```python
from build123d import *

# Parameters (mm, degrees)
SKETCH_1_W          = 20
SKETCH_1_H          = 60
EXTRUDE_1_DEPTH     = 240
SKETCH_2_W          = 14
SKETCH_2_H          = 54
CUT_EXTRUDE_1_DEPTH = 241
SKETCH_3_R          = 2
CUT_EXTRUDE_2_DEPTH = 240
SKETCH_4_R          = 3.05
SKETCH_4_R_2        = 2
CUT_EXTRUDE_3_DEPTH = 61


with BuildPart() as part:
    # 草图1 → 凸台-拉伸1 (new body)
    with BuildSketch(Plane.XY):
        with Locations((-26.616848502, -4.212119477)):
            Rectangle(SKETCH_1_W, SKETCH_1_H)
    extrude(amount=EXTRUDE_1_DEPTH)

    # 草图2 → 切除-拉伸1 (cut, through all)
    with BuildSketch(Plane.XY.offset(240)):
        with Locations((-26.616848502, -4.212119477)):
            Rectangle(SKETCH_2_W, SKETCH_2_H)
    extrude(amount=-CUT_EXTRUDE_1_DEPTH, mode=Mode.SUBTRACT)

    # 草图3 → 切除-拉伸2 (cut)
    with BuildSketch(Plane(origin=(-16.616848502, 0, 0), x_dir=(0, 0, -1), z_dir=(1, 0, 0))):
        with Locations((-220, 19.787880523)):
            Circle(SKETCH_3_R)
        with Locations((-20, 19.787880523)):
            Circle(SKETCH_3_R)
        with Locations((-181.67, 19.787880523)):
            Circle(SKETCH_3_R)
        with Locations((-220, -26.212119477)):
            Circle(SKETCH_3_R)
        with Locations((-181.67, -26.212119477)):
            Circle(SKETCH_3_R)
        with Locations((-20, -26.212119477)):
            Circle(SKETCH_3_R)
        with Locations((-58.33, -26.212119477)):
            Circle(SKETCH_3_R)
        with Locations((-58.33, 19.787880523)):
            Circle(SKETCH_3_R)
    extrude(amount=-CUT_EXTRUDE_2_DEPTH, mode=Mode.SUBTRACT)

    # 草图4 → 切除-拉伸3 (cut, through all)
    with BuildSketch(Plane(origin=(0, 25.787880523, 0), x_dir=(1, 0, 0), z_dir=(0, 1, 0))):
        with Locations((-26.616848502, -220)):
            Circle(SKETCH_4_R)
        with Locations((-26.616848502, -190)):
            Circle(SKETCH_4_R_2)
        with Locations((-26.616848502, -135)):
            Circle(SKETCH_4_R_2)
        with Locations((-26.616848502, -50)):
            Circle(SKETCH_4_R_2)
        with Locations((-26.616848502, -20)):
            Circle(SKETCH_4_R)
        with Locations((-26.616848502, -105)):
            Circle(SKETCH_4_R_2)
    extrude(amount=-CUT_EXTRUDE_3_DEPTH, mode=Mode.SUBTRACT)


solid = part.part
```
Verification items for the finished model (mm, model axes). A direction names the side the tool comes from. Round coordinates to 2 decimals unless told otherwise and drop trailing zeros. Write each loop counter-clockwise with the first axis right and the second up, starting at its lowest first coordinate (ties: lowest second). Pieces come first, ordered by that corner, then holes. Notation, with made-up numbers: (-19.75, 76.25) - (-5.75, 76.25) arc R30 cw to (-5.75, 109.25) - close; hole circle Ø2 at (66, 4). An arc over 180 degrees is marked (long way). Answer as a JSON object with one key per item and string values. Group by question number.
Q1. Thickness scan on line 1 (Y direction, x = -17.5, z = 58.33); line 2 (X direction, y = 20, z = 38); line 3 (X direction, y = 23.75, z = 105). Record the ranges inside material, lowest first.
Q2. Section check C-C, the plane y = 8. Enter the section's corners in (x, z), plus the area to 3 significant figures.
Q3. Mould release check, pull along X, two halves, no side actions. Record for faces 3 (the flat face through (-16.617, -5, 118)), 4 (the flat face through (-27, 25.788, 118)), 5 (the cylindrical face through (-26.877, 24.309, 103.017)), 6 (the flat face through (-27, -31.212, 122)): released by +X, released by -X, zero draft, split by the parting line, or undercut.
Q4. Section check B-B, the plane z = 220. Give the number of separate pieces and of enclosed holes in the cut face, plus the area to 3 significant figures.
Q5. Tool access check on faces 1 (the flat face through (-27, 22.788, 122)), 2 (the cylindrical face through (-35.096, 19.876, 221.998)). Record the directions out of +Z, -Z, +X, -X, +Y, -Y that give a thin tool (end or side, any length) a straight path to the whole face; none if there is none.
Q6. Section check A-A, the plane z = 190. Enter the section's corners in (x, y).
Q7. Go/stop test with a flat-tipped pin: pin 1 Ø4 at (x, y) = (-20, 2) entering from -Z. Record where the tip stops, or that it passes through.
Q8. Section check D-D, the plane z = 115.5. Enter the section's corners in (x, y).
Found:
{
 "1": {"line 1": "y = -34.21 to -28.21, -24.21 to 17.79, 21.79 to 25.79", "line 2": "x = -36.62 to -33.62, -19.62 to -16.62", "line 3": "x = -36.62 to -28.62, -24.62 to -16.62"},
 "2": {"outline": "(-36.62, 0) - (-33.62, 0) - (-33.62, 240) - (-36.62, 240) - close; (-19.62, 0) - (-16.62, 0) - (-16.62, 240) - (-19.62, 240) - close", "area": "1,440 mm^2"},
 "3": {"face 3": "released by +X", "face 4": "zero draft", "face 5": "undercut", "face 6": "undercut"},
 "4": {"separate pieces": "6", "enclosed holes": "0", "area": "359 mm^2"},
 "5": {"face 1": "+Z, -Z", "face 2": "+X, -X"},
 "6": {"outline": "(-36.62, -34.21) - (-28.62, -34.21) - (-28.62, -31.21) - (-33.62, -31.21) - (-33.62, 22.79) - (-28.62, 22.79) - (-28.62, 25.79) - (-36.62, 25.79) - close; (-24.62, -34.21) - (-16.62, -34.21) - (-16.62, 25.79) - (-24.62, 25.79) - (-24.62, 22.79) - (-19.62, 22.79) - (-19.62, -31.21) - (-24.62, -31.21) - close"},
 "7": {"pin 1": "stops at z = 0"},
 "8": {"outline": "(-36.62, -34.21) - (-16.62, -34.21) - (-16.62, 25.79) - (-36.62, 25.79) - close; hole (-33.62, -31.21) - (-19.62, -31.21) - (-19.62, 22.79) - (-33.62, 22.79) - close"}
}
